Part model, mm, in its own coordinate system. A direction names the side the tool comes from. Give positions to 0.01 mm unless a question says otherwise; leave off trailing zeros. Write each loop counter-clockwise with the first axis right and the second up, starting at its lowest first coordinate (ties: lowest second). Pieces come first, ordered by that corner, then holes.
```python
from build123d import *

# Parameters (mm, degrees)
SKETCH1_W           = 27
SKETCH1_H           = 20.2
BOSS_EXTRUDE1_DEPTH = 1.6
SKETCH2_R           = 1
CUT_EXTRUDE1_DEPTH  = 17.935760981
SKETCH4_R           = 0.75
CUT_EXTRUDE2_DEPTH  = 17.935760981
SKETCH6_W           = 6.981427811
SKETCH6_H           = 7.333205182
BOSS_EXTRUDE2_DEPTH = 4
BOSS_EXTRUDE3_DEPTH = 4


with BuildPart() as part:
    # Sketch1 → Boss-Extrude1 (new body)
    with BuildSketch(Plane(origin=(0, 0, 0), x_dir=(1, 0, 0), z_dir=(0, 1, 0))):
        Rectangle(SKETCH1_W, SKETCH1_H)
    extrude(amount=BOSS_EXTRUDE1_DEPTH)

    # Sketch2 → Cut-Extrude1 (cut, through all)
    with BuildSketch(Plane(origin=(0, 1.6, 0), x_dir=(1, 0, 0), z_dir=(0, 1, 0))):
        with Locations(Location((12, 8.310541443, 0), (0, 0, 270))):
            Circle(SKETCH2_R)
        with Locations(Location((12, -8.310541443, 0), (0, 0, 270))):
            Circle(SKETCH2_R)
    extrude(amount=-CUT_EXTRUDE1_DEPTH, mode=Mode.SUBTRACT)

    # Sketch4 → Cut-Extrude2 (cut, through all)
    with BuildSketch(Plane(origin=(0, 1.6, 0), x_dir=(1, 0, 0), z_dir=(0, 1, 0))):
        with Locations(Location((8.835023955, 6.859658721, 0), (0, 0, 270))):
            Circle(SKETCH4_R)
        with Locations(Location((6.295023955, 6.859658721, 0), (0, 0, 270))):
            Circle(SKETCH4_R)
        with Locations(Location((3.755023955, 6.859658721, 0), (0, 0, 270))):
            Circle(SKETCH4_R)
        with Locations(Location((1.215023955, 6.859658721, 0), (0, 0, 270))):
            Circle(SKETCH4_R)
        with Locations(Location((-1.324976045, 6.859658721, 0), (0, 0, 270))):
            Circle(SKETCH4_R)
        with Locations(Location((-3.864976045, 6.859658721, 0), (0, 0, 270))):
            Circle(SKETCH4_R)
    extrude(amount=-CUT_EXTRUDE2_DEPTH, mode=Mode.SUBTRACT)

    # Sketch6 → Boss-Extrude2 (add)
    with BuildSketch(Plane(origin=(0, 1.6, 0), x_dir=(1, 0, 0), z_dir=(0, 1, 0))):
        with Locations((-1.122981606, -4.789584196)):
            Rectangle(SKETCH6_W, SKETCH6_H)
    extrude(amount=BOSS_EXTRUDE2_DEPTH)

    # Sketch7 → Boss-Extrude3 (add)
    with BuildSketch(Plane(origin=(0, 1.6, 0), x_dir=(1, 0, 0), z_dir=(0, 1, 0))):
        with BuildLine():
            Line((-5.758618523, 1.468961855), (-1.736945444, 1.468961855))
            ThreePointArc((-1.736945444, 1.468961855), (-3.747781984, 5.296946033), (-5.758618523, 1.468961855))
        make_face()
    extrude(amount=BOSS_EXTRUDE3_DEPTH)


solid = part.part
```
1) Saw through at A-A, the plane x = 12. Write the cut outline in (y, z).
Answers follow:
outline: (0, -10.1) - (1.6, -10.1) - (1.6, -9.31) - (0, -9.31) - close; (0, -7.31) - (1.6, -7.31) - (1.6, 7.31) - (0, 7.31) - close; (0, 9.31) - (1.6, 9.31) - (1.6, 10.1) - (0, 10.1) - close
2) Pin check, flat tips, straight feed: pin 1 Ø12 at (x, z) = (0, 2.5) entering from -Y; pin 2 Ø1.2 at (x, z) = (8.84, -6.86) entering from +Y; pin 3 Ø1 at (x, z) = (7, 1) entering from +Y; pin 4 Ø1.2 at (x, y) = (-2.5, 3.5) entering from +Z. Stop position of each tip, or through.
Answers follow:
pin 1: stops at y = 0
pin 2: passes through
pin 3: stops at y = 1.6
pin 4: stops at z = 8.46
3) Saw through at C-C, the plane z = 1.75. Write the cut outline in (x, y), then the cut area to 3 significant figures.
Answers follow:
outline: (-13.5, 0) - (13.5, 0) - (13.5, 1.6) - (2.37, 1.6) - (2.37, 5.6) - (-4.61, 5.6) - (-4.61, 1.6) - (-13.5, 1.6) - close
area: 71.1 mm2
4) Saw through at B-B, the plane y = 4.5. Write the cut outline in (x, z).
Answers follow:
outline: (-5.76, -1.47) arc R2.44 ccw (long way) to (-1.74, -1.47) - close; (-4.61, 1.12) - (2.37, 1.12) - (2.37, 8.46) - (-4.61, 8.46) - close
5) Wall check: L1, parallel to Y at x = 4.75, z = -9.5; L2, parallel to X at y = 4.7, z = 6.25; L3, parallel to Z at x = -1, y = 0.75. Give the ranges that are in metal, low to high.
Answers follow:
L1: y = 0 to 1.6
L2: x = -4.61 to 2.37
L3: z = -10.1 to -7.54, -6.18 to 10.1
6) 3-axis set-ups, long thin cutter, end or side, ignore diameter. For faces 5 (the face through (2.368, 4, 5)), 6 (the face through (-3.673, 3.572, -5.296)), 7 (the face through (-1, 4, 8.456)), 8 (the face through (-4.614, 4, 5)), 9 (the face through (0, 1, 10.1)): which of +Z, -Z, +X, -X, +Y, -Y reach the whole face in a straight line?
Answers follow:
face 5: +Z, -Z, +X, +Y
face 6: +Y
face 7: +Z, +X, -X, +Y
face 8: +Z, -X, +Y
face 9: +Z, +X, -X, +Y, -Y
7) Two-plate mould, pull along Z, no slides. Class faces 1 (the face through (0, 1, -10.1)), 2 (the face through (-4, 4, -1.469)), 3 (the face through (8.87, 0.81, -7.61)), 4 (the face through (-1, 5.6, 5)): +Z half, -Z half, draft (parallel to the pull), parting line (faces both ways), or undercut.
Answers follow:
face 1: -Z half
face 2: undercut
face 3: undercut
face 4: draft
8) Saw through at D-D, the plane z = 8. Write the cut outline in (x, y), then the cut area to 3 significant figures.
Answers follow:
outline: (-13.5, 0) - (11.05, 0) - (11.05, 1.6) - (2.37, 1.6) - (2.37, 5.6) - (-4.61, 5.6) - (-4.61, 1.6) - (-13.5, 1.6) - close; (12.95, 0) - (13.5, 0) - (13.5, 1.6) - (12.95, 1.6) - close
area: 68.1 mm2
